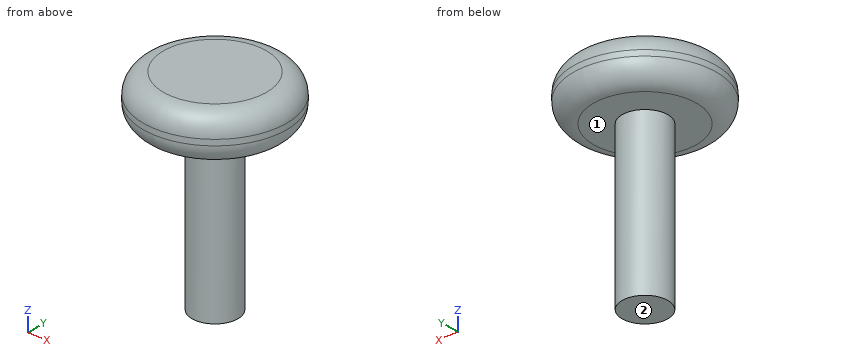
Autodesk Inventor part; units mm, degrees
ref_plane "YZ Plane" through (0, 0, 0) normal (1, 0, 0) x (0, 1, 0)
ref_plane "XZ Plane" through (0, 0, 0) normal (0, 1, 0) x (-1, 0, 0)
ref_plane "XY Plane" through (0, 0, 0) normal (0, 0, 1) x (1, 0, 0)
sketch "Sketch1" plane through (0, 0, 0) normal (0, 0, 1) x (1, 0, 0)
  circle A0 centre (0, 0) radius 4
  dimension "d0" = 8
extrude "Extrusion1" add sketch "Sketch1" along normal blind 28.4
sketch "Sketch2" plane through (0, 0, 28.4) normal (0, 0, 1) x (1, 0, 0)
  circle A0 centre (0, 0) radius 12.5
  dimension "d3" = 25
extrude "Extrusion2" add sketch "Sketch2" along normal blind 8
fillet "Fillet1" radius 3.5 1 edges at (-12.5, 0, 36.4)
fillet "Fillet2" radius 3.5 1 edges at (-12.5, 0, 28.4)
properties part number "Wheel"
For this review, take the finished solid that the model builds, in its own axes (mm). Face numbers are marked on the shaded views. A direction names the side the tool comes from. Coordinates: 2 decimals unless noted, no trailing zeros. Loops run counter-clockwise (first coordinate to the right, second up) from the corner with the lowest first, then second, coordinate; pieces in that order, holes last.
1. Insertion check: P1, Ø1, axis at y = 0.5, z = 6, coming from the +X side; P2, Ø12, axis at x = 8.5, y = 10, coming from the -Z side; P3, Ø12, axis at x = -3, z = 19.5, coming from the +Y side. Each pin has a flat end and moves straight along its axis. Give the tip position at first contact, or say it passes through.
2. Add section A-A, the plane x = 0. Give the boundary of the cut face in (y, z), then the cut area to 3 significant figures.
3. Add section C-C, the plane z = 19.5. Give the boundary of the cut face in (x, y).
4. Add section D-D, the plane z = 31. Give the boundary of the cut face in (x, y), then the cut area to 3 significant figures.
5. For the marked faces 1 and 2, list the 3-axis set-ups (+Z, -Z, +X, -X, +Y, -Y) from which the entire face can be reached by the end or side of a thin tool; tool diameter is ignored.
6. For line 1 (Z direction, x = 6, y = 5.5); line 2 (Z direction, x = 3, y = 11.25); line 3 (X direction, y = -9, z = 33.5), list the stretches that pass through material, from the lowest coordinate up.
Result:
1. P1: stops at x = 4
1. P2: stops at z = 28.4
1. P3: stops at y = 4
2. outline: (-12.5, 31.9) arc R3.5 ccw to (-9, 28.4) - (-4, 28.4) - (-4, 0) - (4, 0) - (4, 28.4) - (9, 28.4) arc R3.5 ccw to (12.5, 31.9) - (12.5, 32.9) arc R3.5 ccw to (9, 36.4) - (-9, 36.4) arc R3.5 ccw to (-12.5, 32.9) - close
2. area: 417 mm2
3. outline: circle Ø8 at (0, 0)
4. outline: circle Ø24.76 at (0, 0)
4. area: 482 mm2
5. face 1: -Z
5. face 2: -Z, +X, -X, +Y, -Y
6. line 1: z = 28.4 to 36.4
6. line 2: z = 29.61 to 35.19
6. line 3: x = -8.6 to 8.6
